Input: part model. Units: mm. Frame: model coordinates. A direction names the side the tool comes from. Give positions to 0.01 mm unless a question says otherwise; leave off trailing zeros. Order: outer loops, then holes, each group sorted by start corner. A loop starts at its lowest first (then second) coordinate and runs counter-clockwise, first axis right, second up. Notation, with made-up numbers: (19, -40) - (41, -40) arc R36 ccw to (41, -2) - close; hole circle Ø5 at (72, 27.5). An arc over 180 degrees is marked (long way). Use a Markdown table: item, result.
from build123d import *

# Parameters (mm, degrees)
CROQUIS1_W              = 40
CROQUIS1_H              = 13
SALIENTE_EXTRUIR1_DEPTH = 13
CROQUIS2_R              = 3.3
CORTAR_EXTRUIR1_DEPTH   = 17
CROQUIS3_R              = 3.2
CORTAR_EXTRUIR4_DEPTH   = 19
CROQUIS7_W              = 17
CROQUIS7_H              = 13
CORTAR_EXTRUIR5_DEPTH   = 9
CROQUIS8_OUTSIDE_W      = 23.804
CROQUIS8_OUTSIDE_H      = 23.804
CROQUIS8_OUTSIDE_R      = 4.2
CORTAR_EXTRUIR6_DEPTH   = 19.1
CROQUIS9_W              = 3.9
CROQUIS9_H              = 13
CORTAR_EXTRUIR7_DEPTH   = 2.3
CROQUIS10_W             = 20.9
CROQUIS10_H             = 13
CORTAR_EXTRUIR8_DEPTH   = 2.3
CORTAR_EXTRUIR9_DEPTH   = 22.3
CORTAR_EXTRUIR10_DEPTH  = 22.3
CORTAR_EXTRUIR11_DEPTH  = 22.3
CORTAR_EXTRUIR12_DEPTH  = 32.3
REDONDEO1_R             = 3


with BuildPart() as part:
    # Croquis1 → Saliente-Extruir1 (new body)
    with BuildSketch(Plane.XY):
        with Locations((20, 6.5)):
            Rectangle(CROQUIS1_W, CROQUIS1_H)
    extrude(amount=SALIENTE_EXTRUIR1_DEPTH)

    # Croquis2 → Cortar-Extruir1 (cut)
    with BuildSketch(Plane(origin=(40, 0, 0), x_dir=(0, 0, -1), z_dir=(1, 0, 0))):
        with Locations((-6.5, 6.5)):
            Circle(CROQUIS2_R)
    extrude(amount=-CORTAR_EXTRUIR1_DEPTH, mode=Mode.SUBTRACT)

    # Croquis3 → Cortar-Extruir4 (cut)
    with BuildSketch(Plane(origin=(0, 13, 0), x_dir=(1, 0, 0), z_dir=(0, 1, 0))):
        with Locations((8, -6.5)):
            Circle(CROQUIS3_R)
    extrude(amount=-CORTAR_EXTRUIR4_DEPTH, mode=Mode.SUBTRACT)

    # Croquis7 → Cortar-Extruir5 (cut)
    with BuildSketch(Plane(origin=(0, 13, 0), x_dir=(1, 0, 0), z_dir=(0, 1, 0))):
        with Locations((8.5, -6.5)):
            Rectangle(CROQUIS7_W, CROQUIS7_H)
    extrude(amount=-CORTAR_EXTRUIR5_DEPTH, mode=Mode.SUBTRACT)

    # Croquis8 outside → Cortar-Extruir6 (cut)
    with BuildSketch(Plane(origin=(40, 0, 0), x_dir=(0, 0, -1), z_dir=(1, 0, 0))):
        with Locations((-6.5, 6.5)):
            Rectangle(CROQUIS8_OUTSIDE_W, CROQUIS8_OUTSIDE_H)
        with Locations((-6.5, 6.5)):
            Circle(CROQUIS8_OUTSIDE_R, mode=Mode.SUBTRACT)
    extrude(amount=-CORTAR_EXTRUIR6_DEPTH, mode=Mode.SUBTRACT)

    # Croquis9 → Cortar-Extruir7 (cut)
    with BuildSketch(Plane(origin=(0, 13, 0), x_dir=(1, 0, 0), z_dir=(0, 1, 0))):
        with Locations((18.95, -6.5)):
            Rectangle(CROQUIS9_W, CROQUIS9_H)
    extrude(amount=-CORTAR_EXTRUIR7_DEPTH, mode=Mode.SUBTRACT)

    # Croquis10 → Cortar-Extruir8 (cut)
    with BuildSketch(Plane.XZ):
        with Locations((10.45, 6.5)):
            Rectangle(CROQUIS10_W, CROQUIS10_H)
    extrude(amount=-CORTAR_EXTRUIR8_DEPTH, mode=Mode.SUBTRACT)

    # Croquis11 → Cortar-Extruir9 (cut)
    with BuildSketch(Plane.XY.offset(13)):
        Polygon((17, 4), (17, 10.7), (20.9, 10.7), align=None)
    extrude(amount=-CORTAR_EXTRUIR9_DEPTH, mode=Mode.SUBTRACT)

    # Croquis13 → Cortar-Extruir10 (cut)
    with BuildSketch(Plane(origin=(20.9, 0, 0), x_dir=(0, 0, -1), z_dir=(1, 0, 0))):
        Polygon((-13, 4), (-13, 10.7), (-8.834314401, 10.7), align=None)
    extrude(amount=-CORTAR_EXTRUIR10_DEPTH, mode=Mode.SUBTRACT)

    # Croquis14 → Cortar-Extruir11 (cut)
    with BuildSketch(Plane(origin=(20.9, 0, 0), x_dir=(0, 0, -1), z_dir=(1, 0, 0))):
        Polygon((0, 4), (0, 10.7), (-4.165524435, 10.7), align=None)
    extrude(amount=-CORTAR_EXTRUIR11_DEPTH, mode=Mode.SUBTRACT)

    # Croquis15 → Cortar-Extruir12 (cut)
    with BuildSketch(Plane(origin=(40, 0, 0), x_dir=(0, 0, -1), z_dir=(1, 0, 0))):
        with BuildLine():
            Line((-10.06680245, 8.717638448), (-11.135301445, 9.381971415))
            ThreePointArc((-11.135301445, 9.381971415), (-6.499952655, 11.958184563), (-1.864648558, 9.381891))
            Line((-1.864648558, 9.381891), (-2.933159079, 8.717576569))
            ThreePointArc((-2.933159079, 8.717576569), (-6.499963568, 10.7), (-10.06680245, 8.717638448))
        make_face()
    extrude(amount=-CORTAR_EXTRUIR12_DEPTH, mode=Mode.SUBTRACT)

    # Redondeo1
    redondeo1_edges = [part.edges().sort_by_distance(p)[0] for p in [
        (0, 3.15, 0),
        (0, 3.15, 13),
    ]]
    fillet(redondeo1_edges, radius=REDONDEO1_R)


solid = part.part
1. Material intervals for line 1 along Y through (x, z) = (26.5, 6.5); line 2 along X through (y, z) = (3.4, 6.5); line 3 along Z through (x, y) = (8, 3.15), sorted ascending.
Response:
| item | result |
|---|---|
| line 1 | y = 2.3 to 3.2, 9.8 to 10.7 |
| line 2 | x = 0 to 4.8, 11.2 to 23 |
| line 3 | z = 0 to 3.3, 9.7 to 13 |
2. Pin query (flat end, axial travel): pin 1 (5 mm diameter, centred on x = 8, z = 11.5, fed in from +Y); pin 2 (5 mm diameter, centred on y = 9, z = 3, fed in from -X); pin 3 (3 mm diameter, centred on x = 11, y = 6, fed in from +Z); pin 4 (2 mm diameter, centred on y = 5.5, z = 5, fed in from +X). Return the tip coordinate at first contact, or that it passes through.
Response:
| item | result |
|---|---|
| pin 1 | stops at y = 4 |
| pin 2 | stops at x = 18.46 |
| pin 3 | passes through |
| pin 4 | stops at x = 23 |
3. Section query D-D (y = 6.5). Return loops of the section in (x, z), then the cut area to 3 significant figures.
Response:
| item | result |
|---|---|
| outline | (18.46, 1.55) - (20.9, 1.55) - (20.9, 2.3) - (40, 2.3) - (40, 3.2) - (23, 3.2) - (23, 9.8) - (40, 9.8) - (40, 10.7) - (20.9, 10.7) - (20.9, 11.45) - (18.46, 11.45) - close |
| area | 72.4 mm^2 |
4. Mould query, pull axis X, two halves, no side actions, for faces 1 (the face through (40, 4, 9)), 2 (the face through (10, 3, 4)), 3 (the face through (18.544, 6.652, 6.591)). Classes: pulls with the +X half, pulls with the -X half, needs draft (parallel to the pull), parting line crosses it, or undercut.
Response:
| item | result |
|---|---|
| face 1 | pulls with the +X half |
| face 2 | undercut |
| face 3 | pulls with the -X half |
5. Set-up query: faces 4 (the face through (12, 3, 13)), 5 (the face through (23, 7, 7)), 6 (the face through (10.3, 4, 3.5)). Return all of +Z, -Z, +X, -X, +Y, -Y with unobstructed straight access to the full face (end or side cutting, diameter ignored); none if empty.
Response:
| item | result |
|---|---|
| face 4 | +Z, +X, -X, +Y, -Y |
| face 5 | +X |
| face 6 | +Z, -Z, -X, +Y |
6. Section query C-C (x = 36.5). Return loops of the section in (y, z), then the cut area to 3 significant figures.
Response:
| item | result |
|---|---|
| outline | circle Ø8.4 at (6.5, 6.5); hole circle Ø6.6 at (6.5, 6.5) |
| area | 21.2 mm^2 |
7. Section query B-B (z = 5.75). Return loops of the section in (x, y).
Response:
| item | result |
|---|---|
| outline | (0, 2.3) - (4.89, 2.3) - (4.89, 4) - (0, 4) - close; (11.11, 2.3) - (20.9, 2.3) - (20.9, 2.37) - (40, 2.37) - (40, 3.29) - (23, 3.29) - (23, 9.71) - (40, 9.71) - (40, 10.63) - (20.86, 10.63) - (17, 4) - (11.11, 4) - close |
8. Section query A-A (x = 8). Return loops of the section in (y, z), then the cut area to 3 significant figures.
Response:
| item | result |
|---|---|
| outline | (2.3, 0) - (4, 0) - (4, 3.3) - (2.3, 3.3) - close; (2.3, 9.7) - (4, 9.7) - (4, 13) - (2.3, 13) - close |
| area | 11.2 mm^2 |
